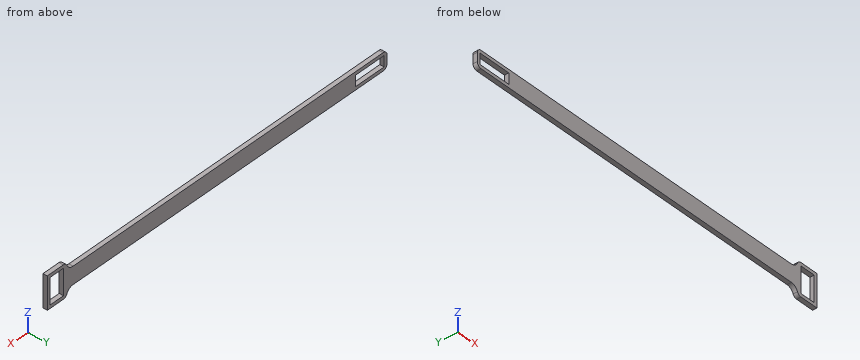
from build123d import *

# Parameters (mm, degrees)
SKETCH1_W           = 7
SKETCH1_H           = 12
SKETCH1_W_2         = 15
SKETCH1_H_2         = 5
BOSS_EXTRUDE1_DEPTH = 2
FILLET1_R           = 2


with BuildPart() as part:
    # Sketch1 → Boss-Extrude1 (new body)
    with BuildSketch(Plane(origin=(0, 0, 0), x_dir=(1, 0, 0), z_dir=(0, 1, 0))):
        with BuildLine():
            Line((-93, 4), (-93, -4))
            Line((-93, -4), (71.500000067, -4))
            ThreePointArc((71.500000067, -4), (73.974873758, -5.025126289), (75, -7.5))
            Line((75, -7.5), (85, -7.5))
            Line((85, -7.5), (85, 7.5))
            Line((85, 7.5), (75, 7.5))
            ThreePointArc((75, 7.5), (73.974873696, 5.025126228), (71.499999892, 4))
            Line((71.499999892, 4), (-93, 4))
        make_face()
        with Locations((80, 0)):
            Rectangle(SKETCH1_W, SKETCH1_H, mode=Mode.SUBTRACT)
        with Locations((-84, 0)):
            Rectangle(SKETCH1_W_2, SKETCH1_H_2, mode=Mode.SUBTRACT)
    extrude(amount=BOSS_EXTRUDE1_DEPTH)

    # Fillet1
    fillet1_edges = [part.edges().sort_by_distance(p)[0] for p in [
        (-93, 1, 4),
        (-93, 1, -4),
        (75, 1, -7.5),
        (75, 1, 7.5),
    ]]
    fillet(fillet1_edges, radius=FILLET1_R)


solid = part.part
Part model, mm, in its own coordinate system. Coordinates: 2 decimals unless noted, no trailing zeros. Loops run counter-clockwise (first coordinate to the right, second up) from the corner with the lowest first, then second, coordinate; pieces in that order, holes last. Notation, with made-up numbers: (75, 49) -> (132, 49) arc R26 ccw to (132, 71) -> close; hole circle Ø5 at (33, 89.5). An arc over 180 degrees is marked (long way). Use a Markdown table: item, result. Add a question column.
Item 1: Band-saw the part on A-A on y = 0.7. Write the cut outline in (x, z).
Item 2: Band-saw the part on B-B on x = 6.5. Write the cut outline in (y, z).
Item 3: Probe probe 1 along X at (y, z) = (1.4, 1.25); probe 2 along Z at (x, y) = (69, 1.8); probe 3 along X at (y, z) = (1.7, 3). List the from-to ranges inside material, lowest first.
Geometry says:
| question | item | result |
|---|---|---|
| 1 | outline | (-93, -2) arc R2 ccw to (-91, -4) -> (71.5, -4) arc R3.5 cw to (74.76, -6.23) arc R2 ccw to (76.62, -7.5) -> (85, -7.5) -> (85, 7.5) -> (76.62, 7.5) arc R2 ccw to (74.76, 6.23) arc R3.5 cw to (71.5, 4) -> (-91, 4) arc R2 ccw to (-93, 2) -> close; hole (-91.5, -2.5) -> (-76.5, -2.5) -> (-76.5, 2.5) -> (-91.5, 2.5) -> close; hole (76.5, -6) -> (83.5, -6) -> (83.5, 6) -> (76.5, 6) -> close |
| 2 | outline | (0, -4) -> (2, -4) -> (2, 4) -> (0, 4) -> close |
| 3 | probe 1 | -93 to -91.5, -76.5 to 76.5, 83.5 to 85 |
| 3 | probe 2 | -4 to 4 |
| 3 | probe 3 | -92.73 to 76.5, 83.5 to 85 |
